CAD build for the part. Positions are in the model's coordinates, mm. Face numbers are marked on the shaded views. A direction names the side the tool comes from. Coordinates: 2 decimals unless noted, no trailing zeros. Loops run counter-clockwise (first coordinate to the right, second up) from the corner with the lowest first, then second, coordinate; pieces in that order, holes last. Notation, with made-up numbers: (-11.75, 34.5) -> (24.25, 34.5) arc R18 ccw to (24.25, 47.5) -> close; hole circle Ø2 at (61.5, 18). An arc over 180 degrees is marked (long way). Return JSON: item names as keys, results as strings. Group by question number.
(1) Flat gauge pins, fed straight in: pin 1 Ø6 at (y, z) = (3.5, -4.5) entering from +X; pin 2 Ø1 at (x, z) = (1, -0.5) entering from -Y; pin 3 Ø2.5 at (y, z) = (-3, 6) entering from -X. Where does each tip first touch, or does it go through?
(2) Tool access for the marked faces 5 and 6: list every direction of +Z, -Z, +X, -X, +Y, -Y with a clear straight run to the whole face (end or side of a thin tool).
(3) Saw through at A-A on z = -4. Write the cut outline in (x, y), then the cut area to 3 significant figures.
(4) Saw through at C-C on x = 1. Write the cut outline in (y, z), then the cut area to 3 significant figures.
(5) Mould opens along Z. For the marked faces 1, 2, 3 and 4 say: pulls with the +Z half, pulls with the -Z half, needs draft (parallel to the pull), parting line crosses it, or undercut.
(6) Probe L1, parallel to Y at x = 1.1, z = 6; L2, parallel to Y at x = 1.4, z = -4; L3, parallel to Z at x = 1, y = 3. List the from-to ranges inside material, lowest first.
(7) Saw through at B-B on y = -3. Write the cut outline in (x, z), then the cut area to 3 significant figures.
```python
from build123d import *

# Parameters (mm, degrees)
EXTRUDE_1_DEPTH            = 2
HOLE_WIZARD_M31_AT_2_COUNT = 2
HOLE_WIZARD_M31_AT_2_PITCH = 11.66190379
CHAMFER_2_SIZE             = 2


with BuildPart() as part:
    # Эскиз1 → Бобышка-Вытянуть1 (new body)
    with BuildSketch(Plane(origin=(0, 0, 0), x_dir=(0, 0, -1), z_dir=(1, 0, 0))):
        Polygon((-9, -6), (-2, -6), (-2, 0), (9, 0), (9, 6), (-9, 6), align=None)
    extrude(amount=EXTRUDE_1_DEPTH)

    # Эскиз2 → Отверстие обработанное метчиком M31 (revolve, cut)
    with BuildSketch(Plane(origin=(2, 3, -4), x_dir=(0, 0, -1), z_dir=(0, 1, 0))):
        Polygon((0, 0), (0, 2), (1.6, 2), (1.5, 1.929979246), (1.5, 0.070020754), (1.6, 0), align=None)
    hole_wizard_m31 = revolve(axis=Axis((8.35, 3, -4), (-1, 0, 0)), mode=Mode.SUBTRACT)

    # Отверстие обработанное метчиком M31 at 2: Отверстие обработанное метчиком M31 ×2
    with Locations(*[Vector(0, -0.514495755, 0.857492926) * (i * HOLE_WIZARD_M31_AT_2_PITCH) for i in range(1, HOLE_WIZARD_M31_AT_2_COUNT)]):
        add(hole_wizard_m31, mode=Mode.SUBTRACT)

    # Фаска2
    chamfer_2_edges = [part.edges().sort_by_distance(p)[0] for p in [
        (1, -6, 9),
    ]]
    chamfer(chamfer_2_edges, length=CHAMFER_2_SIZE)


solid = part.part
```
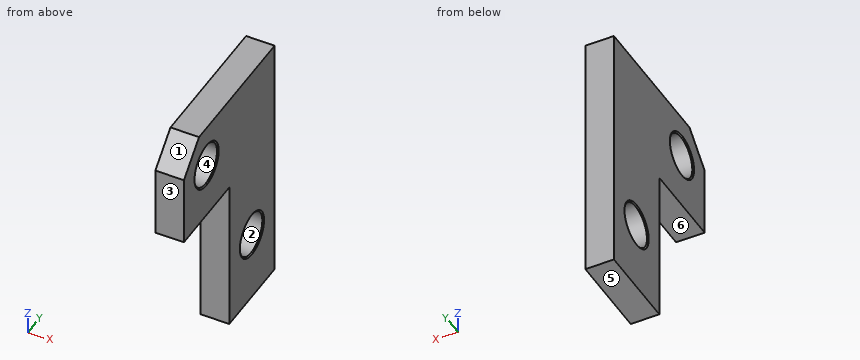
Geometry results:
{
 "1": {"pin 1": "x = 2", "pin 2": "y = 0", "pin 3": "through"},
 "2": {"face 5": "-Z, +X, -X, +Y, -Y", "face 6": "-Z, +X, -X, -Y"},
 "3": {"outline": "(0, 0) -> (2, 0) -> (2, 1.4) -> (1.93, 1.5) -> (0.07, 1.5) -> (0, 1.4) -> close; (0, 4.6) -> (0.07, 4.5) -> (1.93, 4.5) -> (2, 4.6) -> (2, 6) -> (0, 6) -> close", "area": "5.99 mm²"},
 "4": {"outline": "(-6, 2) -> (0, 2) -> (0, -9) -> (6, -9) -> (6, 9) -> (-4, 9) -> (-6, 7) -> close; hole circle Ø3 at (-3, 6); hole circle Ø3 at (3, -4)", "area": "134 mm²"},
 "5": {"face 1": "pulls with the +Z half", "face 2": "undercut", "face 3": "needs draft", "face 4": "undercut"},
 "6": {"L1": "-6 to -4.5, -1.5 to 6", "L2": "0 to 1.5, 4.5 to 6", "L3": "-9 to -5.5, -2.5 to 9"},
 "7": {"outline": "(0, 2) -> (2, 2) -> (2, 4.4) -> (1.93, 4.5) -> (0.07, 4.5) -> (0, 4.4) -> close; (0, 7.6) -> (0.07, 7.5) -> (1.93, 7.5) -> (2, 7.6) -> (2, 9) -> (0, 9) -> close", "area": "7.99 mm²"}
}
